Source: CAD feature listing. Evaluate the final solid. Frame: model axes, mm. A direction names the side the tool comes from. Coordinates: 2 decimals unless noted, no trailing zeros. Loops run counter-clockwise (first coordinate to the right, second up) from the corner with the lowest first, then second, coordinate; pieces in that order, holes last. Notation, with made-up numbers: (78, 75) -> (127, 75) arc R18 cw to (127, 110) -> close; hole circle Ø1 at (-13, -9.5). An arc over 180 degrees is marked (long way). Answer as CSV lines item,"result".
from build123d import *

# Parameters (mm, degrees)
SZKIC1_W                    = 149.6
SZKIC1_H                    = 85.5
SZKIC1_R                    = 2
SZKIC1_W_2                  = 75
SZKIC1_H_2                  = 75
SZKIC1_W_3                  = 50.2
SZKIC1_H_3                  = 22.6
SZKIC1_W_4                  = 21.2
SZKIC1_H_4                  = 16.2
SZKIC1_H_5                  = 20
SZKIC1_R_2                  = 2.25
DODANIE_WYCI_GNI_CIE1_DEPTH = 3
ZAOKR_GLENIE1_R             = 3
ZAOKR_GLENIE2_R             = 3


with BuildPart() as part:
    # Szkic1 → Dodanie-wyciągnięcie1 (new body)
    # profile 1 of 2: a face of its own
    with BuildSketch(Plane.XY):
        with Locations((0.286770428, 26.82962954)):
            Rectangle(SZKIC1_W, SZKIC1_H)
        with Locations((45.086770428, -9.62037046)):
            Circle(SZKIC1_R, mode=Mode.SUBTRACT)
        with Locations((68.786770428, 63.27962954)):
            Circle(SZKIC1_R, mode=Mode.SUBTRACT)
        with Locations((-68.213229572, 0.07962954)):
            Circle(SZKIC1_R, mode=Mode.SUBTRACT)
        with Locations((-68.213229572, 63.27962954)):
            Circle(SZKIC1_R, mode=Mode.SUBTRACT)
        with Locations((-21.013229572, 26.82962954)):
            Rectangle(SZKIC1_W_2, SZKIC1_H_2, mode=Mode.SUBTRACT)
        with Locations((45.086770428, 41.37962954)):
            Rectangle(SZKIC1_W_3, SZKIC1_H_3, mode=Mode.SUBTRACT)
        with Locations((44.586770428, 6.07962954)):
            Rectangle(SZKIC1_W_4, SZKIC1_H_4, mode=Mode.SUBTRACT)
    # profile 2 of 2: a face of its own
    with BuildSketch(Plane.XY):
        with Locations((0.286770428, -25.92037046)):
            Rectangle(SZKIC1_W, SZKIC1_H_5)
        with Locations((65.086770428, -25.92037046)):
            Circle(SZKIC1_R_2, mode=Mode.SUBTRACT)
        with Locations((0.286770428, -25.92037046)):
            Circle(SZKIC1_R_2, mode=Mode.SUBTRACT)
        with Locations((-64.513229572, -25.92037046)):
            Circle(SZKIC1_R_2, mode=Mode.SUBTRACT)
    extrude(amount=DODANIE_WYCI_GNI_CIE1_DEPTH)

    # Zaokrąglenie1
    zaokr_glenie1_edges = [part.edges().sort_by_distance(p)[0] for p in [
        (-58.513229572, 64.32962954, 1.5),
        (-58.513229572, -10.67037046, 1.5),
        (16.486770428, -10.67037046, 1.5),
        (16.486770428, 64.32962954, 1.5),
        (75.086770428, -35.92037046, 1.5),
        (-74.513229572, -35.92037046, 1.5),
        (-74.513229572, 69.57962954, 1.5),
        (75.086770428, 69.57962954, 1.5),
    ]]
    fillet(zaokr_glenie1_edges, radius=ZAOKR_GLENIE1_R)

    # Zaokrąglenie2
    zaokr_glenie2_edges = [part.edges().sort_by_distance(p)[0] for p in [
        (19.986770428, 52.67962954, 1.5),
        (19.986770428, 30.07962954, 1.5),
        (70.186770428, 30.07962954, 1.5),
        (70.186770428, 52.67962954, 1.5),
    ]]
    fillet(zaokr_glenie2_edges, radius=ZAOKR_GLENIE2_R)


solid = part.part
(1) Cut plane D-D (y = 26.5). Return the cut outline in (x, z), then the cut area to 3 significant figures.
Computed values:
outline,"(-74.51, 0) -> (-58.51, 0) -> (-58.51, 3) -> (-74.51, 3) -> close; (16.49, 0) -> (75.09, 0) -> (75.09, 3) -> (16.49, 3) -> close"
area,"224 mm^2"
(2) Cut plane C-C (x = 51). Return the cut outline in (y, z).
Computed values:
outline,"(-35.92, 0) -> (-2.02, 0) -> (-2.02, 3) -> (-35.92, 3) -> close; (14.18, 0) -> (30.08, 0) -> (30.08, 3) -> (14.18, 3) -> close; (52.68, 0) -> (69.58, 0) -> (69.58, 3) -> (52.68, 3) -> close"
(3) Pin query (flat end, axial travel): pin 1 Ø2.5 at (x, y) = (-64.51, -25.92) entering from -Z. Return the tip coordinate at first contact, or that it passes through.
Computed values:
pin 1,"through"
(4) Material intervals for L1, parallel to X at y = 49, z = 0.55; L2, parallel to X at y = -26, z = 2.45; L3, parallel to Y at x = 38, z = 2.3, sorted ascending. Write a range as [from, to].
Computed values:
L1,"[-74.51, -58.51], [16.49, 19.99], [70.19, 75.09]"
L2,"[-74.51, -66.76], [-62.26, -1.96], [2.54, 62.84], [67.34, 75.09]"
L3,"[-35.92, -2.02], [14.18, 30.08], [52.68, 69.58]"
(5) Draft query along X for faces 3 (the cylindrical face through (74.23, 68.68, 1.52)), 4 (the flat face through (33.987, 6, 1)), 5 (the flat face through (-1, -35.92, 1)). Return one class per face: released by +X, released by -X, zero draft, split by the parting line, or undercut.
Computed values:
face 3,"released by +X"
face 4,"undercut"
face 5,"zero draft"
(6) Access query for faces 1 (the flat face through (44, 14.18, 1)), 2 (the flat face through (32, 6, 3)). Directions: +Z, -Z, +X, -X, +Y, -Y. A direction counts if a zero-diameter tool reaches every point of the face in a straight line with its end or side. Return the directions, or none.
Computed values:
face 1,"+Z, -Z"
face 2,"+Z, +X, -X, +Y, -Y"
(7) Cut plane A-A (x = -45.5). Return the cut outline in (y, z).
Computed values:
outline,"(-35.92, 0) -> (-10.67, 0) -> (-10.67, 3) -> (-35.92, 3) -> close; (64.33, 0) -> (69.58, 0) -> (69.58, 3) -> (64.33, 3) -> close"
(8) Cut plane B-B (y = 48). Return the cut outline in (x, z).
Computed values:
outline,"(-74.51, 0) -> (-58.51, 0) -> (-58.51, 3) -> (-74.51, 3) -> close; (16.49, 0) -> (19.99, 0) -> (19.99, 3) -> (16.49, 3) -> close; (70.19, 0) -> (75.09, 0) -> (75.09, 3) -> (70.19, 3) -> close"
